Could you check a few things on this model? Use its own coordinates, in mm. Face numbers are marked on the shaded views. A direction names the side the tool comes from. Coordinates: 2 decimals unless noted, no trailing zeros. Loops run counter-clockwise (first coordinate to the right, second up) from the corner with the lowest first, then second, coordinate; pieces in that order, holes last.
Autodesk Inventor part; units mm, degrees
ref_plane "YZ Plane" through (0, 0, 0) normal (1, 0, 0) x (0, 1, 0)
ref_plane "XZ Plane" through (0, 0, 0) normal (0, 1, 0) x (-1, 0, 0)
ref_plane "XY Plane" through (0, 0, 0) normal (0, 0, 1) x (1, 0, 0)
sketch "Sketch1" plane through (0, 0, 0) normal (0, 1, 0) x (-1, 0, 0)
  circle A0 centre (0, 0) radius 4.05
  line L0 (0, 12.5) -> (150, 12.5)
  arc A1 (150, -12.5) -> (150, 12.5) centre (150, 0) ccw
  line L1 (150, -12.5) -> (0, -12.5)
  arc A2 (0, 12.5) -> (0, -12.5) centre (0, 0) ccw
  dimension "d0" = 150
  dimension "d2" = 12.5
  dimension "d3" = 8.1
extrude "Extrusion1" add sketch "Sketch1" along normal blind 25
sketch "Sketch2" plane through (0, 25, 0) normal (0, 1, 0) x (1, 0, 0)
  circle A0 centre (0, 0) radius 4.05
  line L0 (-150, -12.5) -> (0, -12.5)
  line L1 (0, 12.5) -> (-150, 12.5)
  arc A1 (-150, 12.5) -> (-150, -12.5) centre (-150, 0) ccw
  line L2 (-80, 12.5) -> (-80, -12.5)
  dimension "d6" = 80
extrude "Extrusion2" add sketch "Sketch2" along normal blind 26.5 contours A1 L1 L2 L0
sketch "Sketch3" plane through (-150, 0, 12.5) normal (0, 0, 1) x (1, 0, 0)
  line L0 (150, 0) -> (0, 0)
  line L1 (70, 25) -> (70, 51.5)
  line L2 (0, 51.5) -> (70, 51.5)
  line L3 (70, 25) -> (43.5, 51.5)
  line L4 (59.6447, 0) -> (33.1447, 26.5)
  line L5 (70, 51.5) -> (70, 25)
  line L6 (70, 25) -> (150, 25)
  line L7 (150, 0) -> (150, 25)
  line L8 (150, 0) -> (0, 0)
  line L9 (0, 0) -> (0, 51.5)
  line L10 (-12.5, 0) -> (-12.5, 51.5)
  line L11 (-12.5, 26.5) -> (33.1447, 26.5)
  line L12 (-12.5, 26.5) -> (-12.5, 0)
  line L13 (59.6447, 0) -> (-12.5, 0)
  line L14 (0, 51.5) -> (70, 51.5)
  dimension "d9" = 45
  dimension "d10" = 25
  dimension "d11" = 25
extrude "Extrusion3" cut sketch "Sketch3" against normal through all contours L0 L9 L11 L4 | L13 L10 L11 L9
sketch "Sketch4" plane through (0, 0, 12.5) normal (0, 0, 1) x (1, 0, 0)
  line L0 (-116.8553, 26.5) -> (-90.3553, 0)
  line L1 (-80, 25) -> (-80, 51.5)
  line L2 (-150, 51.5) -> (-80, 51.5)
  line L3 (-80, 25) -> (-106.5, 51.5)
extrude "Extrusion4" cut sketch "Sketch4" against normal through all
sketch "Sketch5" plane through (0, 51.5, 0) normal (0, 1, 0) x (1, 0, 0)
  arc A0 (-150, 12.5) -> (-150, -12.5) centre (-150, 0) ccw
  circle A1 centre (-150, 0) radius 8.3
  point P0 (0, 0)
  dimension "d20" = 16.6
extrude "Extrusion5" cut sketch "Sketch5" against normal through all
sketch "Sketch6" plane through (0, 51.5, 0) normal (0, 1, 0) x (1, 0, 0)
  circle A0 centre (-150, 0) radius 8.3
  arc A1 (-150, 12.5) -> (-150, -12.5) centre (-150, 0) ccw
  circle A2 centre (-150, 0) radius 10.55
  point P0 (0, 0)
  dimension "d26" = 21.1
extrude "Extrusion6" cut sketch "Sketch6" against normal blind 4
sketch "Sketch7" plane through (-150, 26.5, 12.5) normal (0, -1, 0) x (1, 0, 0)
  circle A0 centre (0, -12.5) radius 8.3
  circle A1 centre (0, -12.5) radius 10.55
  point P0 (150, -12.5)
extrude "Extrusion7" cut sketch "Sketch7" against normal blind 4
sketch "Sketch8" plane through (0, 51.5, 0) normal (0, 1, 0) x (1, 0, 0)
  circle A0 centre (-150, 0) radius 10.55
  arc A1 (-150, 12.5) -> (-150, -12.5) centre (-150, 0) ccw
  circle A2 centre (-150, 0) radius 13.55
  point P0 (0, 0)
  dimension "d32" = 3
extrude "Extrusion8" add sketch "Sketch8" against normal up to surface (25 mm away)
sketch "Sketch9" plane through (0, 0, 0) normal (0, -1, 0) x (1, 0, 0)
  line L0 (0, 12.5) -> (-90.3553, 12.5)
  circle A0 centre (0, 0) radius 4.05
  line L1 (0, 0) -> (-25, 0)
  circle A1 centre (-25, 0) radius 1.5
  dimension "d35" = 25
  dimension "d36" = 3
extrude "Extrusion9" cut sketch "Sketch9" against normal through all contours A1
sketch "Sketch14" plane through (0, 51.5, 0) normal (0, 1, 0) x (1, 0, 0)
  line L0 (-106.5, 12.5) -> (-144.77, 12.5)
  arc A0 (-144.77, 12.5) -> (-144.77, -12.5) centre (-150, 0) ccw
  line L1 (-144.77, -12.5) -> (-155.23, -12.5)
  point P0 (0, 0)
sketch "Sketch15" plane through (0, 51.5, 0) normal (0, 1, 0) x (1, 0, 0)
  line L0 (-106.5, 12.5) -> (-144.77, 12.5)
  arc A0 (-144.77, 12.5) -> (-155.23, -12.5) centre (-150, 0) ccw
  line L1 (-155.23, -12.5) -> (-158.4293, -12.5)
  line L2 (-158.4293, -12.5) -> (-161.7346, -6.775)
  point P0 (0, 0)
  dimension "d52" = 120
sketch "Sketch16" plane through (0, 25, 0) normal (0, 1, 0) x (1, 0, 0)
  arc A0 (0, -12.5) -> (0, 12.5) centre (0, 0) ccw
  line L0 (0, 12.5) -> (-80, 12.5)
  line L1 (0, -12.5) -> (7.2169, -12.5)
  line L2 (7.2169, -12.5) -> (10.8253, -6.25)
  dimension "d55" = 120
properties part number "xy forearm"
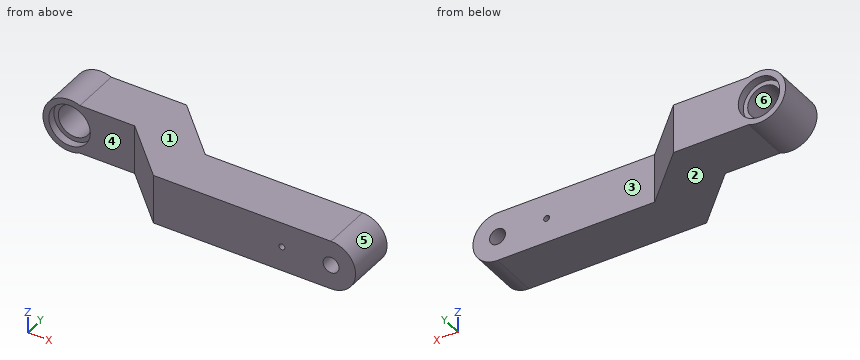
(1) Imagine slicing it at A-A, the plane x = -150. Write out the boundary of the cut face in (y, z), and give its area (4 significant figures).
Answers:
outline: (26.5, -13.55) - (51.5, -13.55) - (51.5, -10.55) - (47.5, -10.55) - (47.5, -8.3) - (30.5, -8.3) - (30.5, -10.55) - (26.5, -10.55) - close; (26.5, 10.55) - (30.5, 10.55) - (30.5, 8.3) - (47.5, 8.3) - (47.5, 10.55) - (51.5, 10.55) - (51.5, 13.55) - (26.5, 13.55) - close
area: 226.5 mm2
(2) Imagine slicing it at B-B, the plane y = 34.5. Write out the boundary of the cut face in (x, z), and give its area (3 significant figures).
Answers:
outline: (-144.77, -12.5) - (-89.5, -12.5) - (-89.5, 12.5) - (-144.77, 12.5) arc R13.55 ccw (long way) to start; hole circle Ø16.6 at (-150, 0)
area: 1,590 mm2
(3) Imagine slicing it at C-C, the plane z = 0. Write out the boundary of the cut face in (x, y).
Answers:
outline: (-163.55, 26.5) - (-160.55, 26.5) - (-160.55, 30.5) - (-158.3, 30.5) - (-158.3, 47.5) - (-160.55, 47.5) - (-160.55, 51.5) - (-163.55, 51.5) - close; (-141.7, 30.5) - (-139.45, 30.5) - (-139.45, 26.5) - (-116.86, 26.5) - (-90.36, 0) - (-26.5, 0) - (-26.5, 25) - (-80, 25) - (-106.5, 51.5) - (-139.45, 51.5) - (-139.45, 47.5) - (-141.7, 47.5) - close; (-23.5, 0) - (-4.05, 0) - (-4.05, 25) - (-23.5, 25) - close; (4.05, 0) - (12.5, 0) - (12.5, 25) - (4.05, 25) - close
(4) I need wall thicknesses on probe 1 along Z at (x, y) = (-150, 27.6); probe 2 along Z at (x, y) = (-150, 36.5); probe 3 along Y at (x, z) = (-118.5, 5.5). Which ranges of each line are inside material? Lowest first, please.
Answers:
probe 1: z = -13.55 to -10.55, 10.55 to 13.55
probe 2: z = -13.55 to -8.3, 8.3 to 13.55
probe 3: y = 26.5 to 51.5
(5) Imagine slicing it at D-D, the plane x = -25. Write out the boundary of the cut face in (y, z).
Answers:
outline: (0, -12.5) - (25, -12.5) - (25, -1.5) - (0, -1.5) - close; (0, 1.5) - (25, 1.5) - (25, 12.5) - (0, 12.5) - close
(6) Which directions (+Z, -Z, +X, -X, +Y, -Y) give clear straight access to the entire face, cutting with the end or side of a thin tool? Please do the marked faces 1, 2 and 3.
Answers:
face 1: +Z, +X, +Y, -Y
face 2: -Z, +X, +Y, -Y
face 3: +Z, -Z, +X, +Y
(7) We'd pull the mould along X, two halves only. Please class the marked faces 4, 5 and 6: +X half, -X half, draft (parallel to the pull), parting line (faces both ways), or undercut.
Answers:
face 4: draft
face 5: +X half
face 6: undercut
(8) For pin 1 (1 mm diameter, centred on y = 17.5, z = 7, fed in from -X); pin 2 (12 mm diameter, centred on y = 12.5, z = 10.5, fed in from +X); pin 3 (3 mm diameter, centred on x = -39, z = -5.5, fed in from +Y), each with a flat end and sliding along its axis, tell me the tip position at first contact or that it passes through.
Answers:
pin 1: stops at x = -108.36
pin 2: stops at x = 11.66
pin 3: stops at y = 25
